Can you work these out from the model? Positions are in its coordinate system, mm. A direction names the side the tool comes from. Give positions to 0.01 mm unless a question says otherwise; leave off trailing zeros. Order: outer loops, then holes, each group sorted by start corner. A loop starts at its lowest first (then second) coordinate and runs counter-clockwise, first axis right, second up. Notation, with made-up numbers: (12.25, 80.5) -> (26.25, 80.5) arc R7 ccw to (26.25, 84.5) -> close; hole circle Ø9 at (28.5, -14). An arc over 180 degrees is marked (long way). Answer as CSV lines item,"result".
```python
from build123d import *

# Parameters (mm, degrees)
SKETCH1_R           = 45
SKETCH1_R_2         = 2
SKETCH1_W           = 20.2
SKETCH1_H           = 40.5
BOSS_EXTRUDE1_DEPTH = 5
CUT_EXTRUDE1_DEPTH  = 10


with BuildPart() as part:
    # Sketch1 → Boss-Extrude1 (new body)
    with BuildSketch(Plane.XY):
        Circle(SKETCH1_R)
        with Locations((0, 42.5)):
            Circle(SKETCH1_R_2, mode=Mode.SUBTRACT)
        with Locations((-42.5, 0)):
            Circle(SKETCH1_R_2, mode=Mode.SUBTRACT)
        with Locations((0, -42.5)):
            Circle(SKETCH1_R_2, mode=Mode.SUBTRACT)
        with Locations((42.5, 0)):
            Circle(SKETCH1_R_2, mode=Mode.SUBTRACT)
        with Locations((-5, -13.85)):
            Circle(SKETCH1_R_2, mode=Mode.SUBTRACT)
        with Locations((5, -13.85)):
            Circle(SKETCH1_R_2, mode=Mode.SUBTRACT)
        with Locations((5, 34.15)):
            Circle(SKETCH1_R_2, mode=Mode.SUBTRACT)
        with Locations((-5, 34.15)):
            Circle(SKETCH1_R_2, mode=Mode.SUBTRACT)
        with Locations((0, 10.15)):
            Rectangle(SKETCH1_W, SKETCH1_H, mode=Mode.SUBTRACT)
    extrude(amount=BOSS_EXTRUDE1_DEPTH)

    # Sketch2 → Cut-Extrude1 (cut)
    with BuildSketch(Plane(origin=(0, 0, 0), x_dir=(-1, 0, 0), z_dir=(0, 0, -1))):
        with BuildLine():
            Line((-19, 18), (-19, -8))
            ThreePointArc((-19, -8), (-23, -12), (-27, -8))
            Line((-27, -8), (-27, 18))
            ThreePointArc((-27, 18), (-23, 22), (-19, 18))
        make_face()
    extrude(amount=-CUT_EXTRUDE1_DEPTH, mode=Mode.SUBTRACT)


solid = part.part
```
Item 1: Imagine slicing it at D-D, the plane y = -13.85. Please give me the cut outline in (x, z).
Numbers:
outline,"(-42.82, 0) -> (-7, 0) -> (-7, 5) -> (-42.82, 5) -> close; (-3, 0) -> (3, 0) -> (3, 5) -> (-3, 5) -> close; (7, 0) -> (42.82, 0) -> (42.82, 5) -> (7, 5) -> close"
Item 2: For faces 4 (the flat face through (-11, 1, 5)), 5 (the cylindrical face through (23, 22, 2)), which set-ups out of +Z, -Z, +X, -X, +Y, -Y let a thin tool reach every point of the face, with its end or its side?
Numbers:
face 4,"+Z, +X, -X, +Y, -Y"
face 5,"+Z, -Z"
Item 3: We'd pull the mould along Y, two halves only. Please class faces 1 (the flat face through (19, 5, 2)), 2 (the flat face through (-11, 1, 0)), 3 (the cylindrical face through (20.765, -39.923, 2.465)): released by +Y, released by -Y, zero draft, split by the parting line, or undercut.
Numbers:
face 1,"undercut"
face 2,"zero draft"
face 3,"split by the parting line"
Item 4: Imagine slicing it at A-A, the plane y = 0. Please give me the cut outline in (x, z), then the cut area to 3 significant figures.
Numbers:
outline,"(-45, 0) -> (-44.5, 0) -> (-44.5, 5) -> (-45, 5) -> close; (-40.5, 0) -> (-10.1, 0) -> (-10.1, 5) -> (-40.5, 5) -> close; (10.1, 0) -> (19, 0) -> (19, 5) -> (10.1, 5) -> close; (27, 0) -> (40.5, 0) -> (40.5, 5) -> (27, 5) -> close; (44.5, 0) -> (45, 0) -> (45, 5) -> (44.5, 5) -> close"
area,"269 mm²"
Item 5: Imagine slicing it at B-B, the plane z = 2.5. Give the number of separate pieces and of enclosed holes in the cut face, then the cut area to 3 significant figures.
Numbers:
separate pieces,"1"
enclosed holes,"10"
area,"5,180 mm²"
Item 6: Please list where these lines run through material, in increasing order: line 1 along Y through (x, z) = (0, 2.7); line 2 along X through (y, z) = (0.5, 3.45); line 3 along Y through (x, z) = (-5, 3.7).
Numbers:
line 1,"y = -45 to -44.5, -40.5 to -10.1, 30.4 to 40.5, 44.5 to 45"
line 2,"x = -45 to -44.44, -40.56 to -10.1, 10.1 to 19, 27 to 40.56, 44.44 to 45"
line 3,"y = -44.72 to -15.85, -11.85 to -10.1, 30.4 to 32.15, 36.15 to 44.72"
Item 7: For pin 1 (8 mm diameter, centred on x = -8.5, y = -6.5, fed in from +Z); pin 2 (3.5 mm diameter, centred on x = 5, y = -13.85, fed in from +Z); pin 3 (2.5 mm diameter, centred on y = 17.5, z = 2, fed in from -X); pin 4 (2 mm diameter, centred on x = -19, z = 3.5, fed in from +Y), each with a flat end and sliding along its axis, tell me the tip position at first contact or that it passes through.
Numbers:
pin 1,"stops at z = 5"
pin 2,"passes through"
pin 3,"stops at x = -41.96"
pin 4,"stops at y = 41.24"
Item 8: Imagine slicing it at C-C, the plane x = 5.5. Please give me the cut outline in (y, z).
Numbers:
outline,"(-44.66, 0) -> (-15.79, 0) -> (-15.79, 5) -> (-44.66, 5) -> close; (-11.91, 0) -> (-10.1, 0) -> (-10.1, 5) -> (-11.91, 5) -> close; (30.4, 0) -> (32.21, 0) -> (32.21, 5) -> (30.4, 5) -> close; (36.09, 0) -> (44.66, 0) -> (44.66, 5) -> (36.09, 5) -> close"
